Work out the finished part from the listing and answer in its coordinate system (mm). Coordinates: 2 decimals unless noted, no trailing zeros. Order: outer loops, then holes, each group sorted by start corner. A loop starts at its lowest first (then second) coordinate and runs counter-clockwise, first axis right, second up.
```python
from build123d import *

# Parameters (mm, degrees)
BOSS_EXTRUDE1_DEPTH = 23.8252
FILLET1_R           = 1.6002


with BuildPart() as part:
    # Sketch1 → Boss-Extrude1 (new body)
    with BuildSketch(Plane(origin=(0, 0, 0), x_dir=(1, 0, 0), z_dir=(0, 1, 0))):
        with BuildLine():
            Line((-34.407907286, 50.8), (34.407907286, 50.8))
            ThreePointArc((34.407907286, 50.8), (35.941054018, 51.941832093), (35.286229068, 53.737806402))
            ThreePointArc((35.286229068, 53.737806402), (0, 64.2874), (-35.286229068, 53.737806402))
            ThreePointArc((-35.286229068, 53.737806402), (-35.941054018, 51.941832093), (-34.407907286, 50.8))
        make_face()
    extrude(amount=BOSS_EXTRUDE1_DEPTH)

    # Fillet1
    fillet1_edges = [part.edges().sort_by_distance(p)[0] for p in [
        (-35.941054018, 23.8252, -51.941832093),
        (0, 23.8252, -50.8),
        (35.941054018, 23.8252, -51.941832093),
        (0, 0, -50.8),
        (-35.941054018, 0, -51.941832093),
        (0, 0, -64.2874),
        (35.941054018, 0, -51.941832093),
        (0, 23.8252, -64.2874),
    ]]
    fillet(fillet1_edges, radius=FILLET1_R)


solid = part.part
```
1. The part is cut by section A-A (y = 16). Determine the outline of the cut face in (x, z), plus the area to 3 significant figures.
2. Flat-ended cylindrical pins translate along their axes: pin 1 (2 mm diameter, centred on x = 20.5, z = -60.5, fed in from -Y); pin 2 (1.5 mm diameter, centred on y = 16, z = -56.5, fed in from -X); pin 3 (1.5 mm diameter, centred on y = 19.5, z = -59.5, fed in from -X). Find the tip coordinate at first contact, or state that the pin passes through.
3. Consider probe 1 along Y at (x, z) = (-30, -55.25); probe 2 along X at (y, z) = (11.25, -55.5); probe 3 along Z at (x, y) = (-3.5, 17.5). Determine where each line is inside the solid, lowest interval first.
Worked out:
1. outline: (-35.29, -53.74) arc R64.29 ccw to (35.29, -53.74) arc R1.6 ccw to (34.41, -50.8) - (-34.41, -50.8) arc R1.6 ccw to start
1. area: 715 mm2
2. pin 1: stops at y = 0.01
2. pin 2: stops at x = -32.01
2. pin 3: stops at x = -26.1
3. probe 1: y = 0.01 to 23.81
3. probe 2: x = -32.44 to 32.44
3. probe 3: z = -64.19 to -50.8
